from build123d import *


with BuildPart() as f1:
    # F0 (on Right) → F1 (revolve)
    with BuildSketch(Plane.YZ):
        Polygon((0, 10.57275), (0, 1.27), (1.5875, 1.27), (1.5875, 0), (2.8575, 0), (2.8575, 0.79375), (2.219446, 3.175), (0.79375, 3.175), (0.79375, 6.604), (3.1115, 6.604), (3.1115, 7.39775), (2.8575, 7.39775), (2.8575, 10.57275), align=None)
    revolve(axis=Axis((0, 0, 5.286375), (0, 0, 1)))


solid = f1.part
The model under review builds one solid part; all positions refer to its coordinate system, in mm. A direction names the side the tool comes from. Give positions to 0.01 mm unless a question says otherwise; leave off trailing zeros. Order: outer loops, then holes, each group sorted by start corner. A loop starts at its lowest first (then second) coordinate and runs counter-clockwise, first axis right, second up. Notation, with made-up numbers: M 59.25,76.5 L 111.25,76.5 A19 cw 111.25,88.5 Z; hole C -10.75,78.5 d8. An arc over 180 degrees is marked long. One line per question, with ' | ' between items. Start each with the question number.
1) Wall thickness on L1, parallel to Z at x = -1.5, y = -1 (3 decimals); L2, parallel to Z at x = 0.5, y = 1 (3 decimals); L3, parallel to Z at x = -0.5, y = 0.25: over which ranges is each line inside the solid? List them lowest first. Write a range as from..to.
2) Consider section C-C, the plane z = 8.75. Give the boundary of the cut face in (x, y) (1 decimal), then the cut area to 3 significant figures.
3) For faces 1 (the face through (-0.858, 2.726, 0.402)), 2 (the face through (-0.858, 2.726, 9.007)), 3 (the face through (1.23, -1.23, 0)), 4 (the face through (0, 1, 3.175)), list the 3-axis set-ups (+Z, -Z, +X, -X, +Y, -Y) from which the entire face can be reached by the end or side of a thin tool; tool diameter is ignored.
4) Consider section D-D, the plane z = 3.75. Give the boundary of the cut face in (x, y).
5) Mouldability with a two-part tool opening along Z and no side actions: class faces 5 (the face through (3.04, -0.67, 7.01)), 6 (the face through (0, 0, 1.27)), 7 (the face through (0.775, -0.172, 4.914)), 8 (the face through (2.335, -0.519, 2.53)) as pulls with the +Z half, pulls with the -Z half, needs draft (parallel to the pull), parting line crosses it, or undercut.
Found:
1) L1: z = 0..3.175, 6.604..10.573 | L2: z = 1.27..3.175, 6.604..10.573 | L3: z = 1.27..10.57
2) outline: C 0,0 d5.7 | area: 25.7 mm²
3) face 1: -Z | face 2: +Z | face 3: -Z, +X, -X, +Y, -Y | face 4: none
4) outline: C 0,0 d1.59
5) face 5: needs draft | face 6: pulls with the -Z half | face 7: undercut | face 8: undercut
